Read the model definition and answer for the solid it produces. Units are mm, in the model's axes. A direction names the side the tool comes from. Give positions to 0.01 mm unless a question says otherwise; leave off trailing zeros. Order: outer loops, then holes, each group sorted by start corner. A loop starts at its lowest first (then second) coordinate and runs counter-clockwise, first axis right, second up. Notation, with made-up numbers: (-3.75, 20.5) - (23.25, 20.5) arc R28 ccw to (23.25, 54.5) - close; hole circle Ø9 at (17.25, 13.25). An arc over 180 degrees is marked (long way). Use a Markdown table: item, result. Add a question column.
1. For a pull along Y with two mould halves and no side action, classify faces 1 (the cylindrical face through (5.56, 2.25, 3.7)), 2 (the cylindrical face through (-0.7, 10.84, 3.8)), 3 (the flat face through (-0.6, 2.3, 0)) as released by +Y, released by -Y, zero draft, split by the parting line, or undercut.
2. A cutting plane is placed at A-A on y = 0. Determine the outline of the cut face in (x, z).
3. Consider L1, parallel to X at y = 0, z = 5.5; L2, parallel to Y at x = 0, z = 4.5; L3, parallel to X at y = 3, z = 4. Determine where each line is inside the solid, lowest interval first.
4. Flat-ended cylindrical pins translate along their axes: P1, Ø1, axis at x = 4.5, z = 1, coming from the -Y side; P2, Ø1.3, axis at y = 3.5, z = 1.5, coming from the +X side; P3, Ø0.6, axis at x = -2, z = 1.5, coming from the -Y side. Find the tip coordinate at first contact, or state that the pin passes through.
5. Which of the six approach directions +Z, -Z, +X, -X, +Y, -Y give full straight-line access (tool end or side, diameter ignored) to faces 4 (the cylindrical face through (0, 4, 4)), 5 (the flat face through (4.287, -5.744, 3.698)), 6 (the flat face through (-2, 2, 1)), 7 (the flat face through (6.349, -5.162, 3.698)), 8 (the flat face through (1, 8, 4))?
6. A cutting plane is placed at C-C on y = 3.25. Determine the outline of the cut face in (x, z), and give its area (3 significant figures).
7. A cutting plane is placed at B-B on x = -3.75. Determine the outline of the cut face in (y, z), and give its area (3 significant figures).
```python
from build123d import *

# Parameters (mm, degrees)
BOSS_EXTRUDE1_DEPTH = 7.5
FILLET1_R           = 1
BOSS_EXTRUDE2_DEPTH = 2
FILLET2_R           = 0.2


with BuildPart() as part:
    # Sketch1 → Boss-Extrude1 (new body)
    with BuildSketch(Plane.XY):
        with BuildLine():
            Line((2.392596776, -3.20553906), (6.280566538, -8.414540033))
            Line((6.280566538, -8.414540033), (7.883336068, -7.218241645))
            Line((7.883336068, -7.218241645), (4.98641234, -3.337018425))
            ThreePointArc((4.98641234, -3.337018425), (5.510375649, 2.373975613), (1, 5.916079783))
            Line((1, 5.916079783), (1, 11.127644916))
            Line((1, 11.127644916), (-1, 11.127644916))
            Line((-1, 11.127644916), (-1, 5.916079783))
            ThreePointArc((-1, 5.916079783), (-5.510375649, 2.373975613), (-4.98641234, -3.337018425))
            Line((-4.98641234, -3.337018425), (-7.883336068, -7.218241645))
            Line((-7.883336068, -7.218241645), (-6.280566538, -8.414540033))
            Line((-6.280566538, -8.414540033), (-2.392596776, -3.20553906))
            ThreePointArc((-2.392596776, -3.20553906), (0, 4), (2.392596776, -3.20553906))
        make_face()
    extrude(amount=BOSS_EXTRUDE1_DEPTH)

    # Fillet1
    fillet1_edges = [part.edges().sort_by_distance(p)[0] for p in [
        (6.280566538, -8.414540033, 3.75),
        (7.883336068, -7.218241645, 3.75),
        (-6.280566538, -8.414540033, 3.75),
        (-7.883336068, -7.218241645, 3.75),
        (-4.98641234, -3.337018425, 3.75),
        (2.392596776, -3.20553906, 3.75),
        (-2.392596776, -3.20553906, 3.75),
        (4.98641234, -3.337018425, 3.75),
        (-1, 5.916079783, 3.75),
        (-1, 11.127644916, 3.75),
        (1, 11.127644916, 3.75),
        (1, 5.916079783, 3.75),
    ]]
    fillet(fillet1_edges, radius=FILLET1_R - 0.0001)  # a hair under: the kernel refuses the full size

    # Sketch2 → Boss-Extrude2 (add)
    with BuildSketch(Plane(origin=(0, 0, 0), x_dir=(-1, 0, 0), z_dir=(0, 0, -1))):
        with BuildLine():
            ThreePointArc((-0.2, 3.994996871), (-2.086004144, 3.413002594), (-3.464101615, 2))
            Line((-3.464101615, 2), (-0.2, 2))
            Line((-0.2, 2), (-0.2, 3.994996871))
        make_face()
        with BuildLine():
            Line((0.2, 3.994996871), (0.2, 2))
            Line((0.2, 2), (3.464101615, 2))
            ThreePointArc((3.464101615, 2), (2.086004144, 3.413002594), (0.2, 3.994996871))
        make_face()
    extrude(amount=-BOSS_EXTRUDE2_DEPTH)

    # Fillet2
    fillet2_edges = [part.edges().sort_by_distance(p)[0] for p in [
        (0.2, 3.994996871, 1),
        (-0.2, 3.994996871, 1),
        (-0.2, 2, 1),
        (0.2, 2, 1),
    ]]
    fillet(fillet2_edges, radius=FILLET2_R - 0.0001)  # a hair under: the kernel refuses the full size


solid = part.part
```
Output values:
| question | item | result |
|---|---|---|
| 1 | face 1 | undercut |
| 1 | face 2 | released by +Y |
| 1 | face 3 | zero draft |
| 2 | outline | (-6, 0) - (-4, 0) - (-4, 7.5) - (-6, 7.5) - close; (4, 0) - (6, 0) - (6, 7.5) - (4, 7.5) - close |
| 3 | L1 | -6 to -4, 4 to 6 |
| 3 | L2 | 4 to 11.13 |
| 3 | L3 | -5.2 to -2.65, 2.65 to 5.2 |
| 4 | P1 | y = -6.7 |
| 4 | P2 | x = 5.28 |
| 4 | P3 | y = 2 |
| 5 | face 4 | +Z |
| 5 | face 5 | +Z, -Z, -Y |
| 5 | face 6 | +Z, -Z |
| 5 | face 7 | +Z, -Z, +X |
| 5 | face 8 | +Z, -Z, +X, +Y |
| 6 | outline | (-5.04, 0) - (-0.2, 0) - (-0.2, 2) - (-2.33, 2) - (-2.33, 7.5) - (-5.04, 7.5) - close; (0.2, 0) - (5.04, 0) - (5.04, 7.5) - (2.33, 7.5) - (2.33, 2) - (0.2, 2) - close |
| 6 | area | 49.2 mm² |
| 7 | outline | (-5.02, 0) - (-1.39, 0) - (-1.39, 7.5) - (-5.02, 7.5) - close; (1.39, 0) - (4.68, 0) - (4.68, 7.5) - (1.39, 7.5) - close |
| 7 | area | 51.9 mm² |
